Input: part model. Units: mm. Frame: model coordinates. A direction names the side the tool comes from. Round coordinates to 2 decimals unless told otherwise and drop trailing zeros. Loops run counter-clockwise (first coordinate to the right, second up) from the corner with the lowest first, then second, coordinate; pieces in that order, holes last. Notation, with made-up numbers: (-11.5, 87) - (24.5, 87) arc R22 ccw to (24.5, 99) - close; hole circle Ø1 at (57.25, 41.5). An arc over 180 degrees is marked (long way). One line per question, with ' | ' between items. Start each with the question number.
from build123d import *

# Parameters (mm, degrees)
SKETCH1_R           = 6.35
SKETCH1_R_2         = 1.905
SKETCH1_R_3         = 11.43
BOSS_EXTRUDE1_DEPTH = 10.16
SKETCH8_R           = 6.35
CUT_EXTRUDE3_DEPTH  = 9.398
FILLET1_R           = 6.35
FILLET3_R           = 2.54


with BuildPart() as part:
    # Sketch1 → Boss-Extrude1 (new body)
    with BuildSketch(Plane(origin=(0, 0, 0), x_dir=(1, 0, 0), z_dir=(0, 1, 0))):
        with BuildLine():
            ThreePointArc((54.61, -31.75), (22.86, 0), (54.61, 31.75))
            Line((54.61, 31.75), (69.270321928, 31.75))
            ThreePointArc((69.270321928, 31.75), (-76.2, 0), (69.270321928, -31.75))
            Line((69.270321928, -31.75), (54.61, -31.75))
        make_face()
        with Locations(Location((0, -60.96, 0), (0, 0, 270))):
            Circle(SKETCH1_R, mode=Mode.SUBTRACT)
        with Locations(Location((-15.499999988, -15.499999988, 0), (0, 0, 270))):
            Circle(SKETCH1_R_2, mode=Mode.SUBTRACT)
        with Locations(Location((15.499999988, -15.499999988, 0), (0, 0, 270))):
            Circle(SKETCH1_R_2, mode=Mode.SUBTRACT)
        with Locations(Location((-15.499999988, 15.499999988, 0), (0, 0, 270))):
            Circle(SKETCH1_R_2, mode=Mode.SUBTRACT)
        with Locations(Location((0, 0, 0), (0, 0, 270))):
            Circle(SKETCH1_R_3, mode=Mode.SUBTRACT)
        with Locations(Location((15.499999988, 15.499999988, 0), (0, 0, 270))):
            Circle(SKETCH1_R_2, mode=Mode.SUBTRACT)
    extrude(amount=BOSS_EXTRUDE1_DEPTH)

    # Sketch8 → Cut-Extrude3 (cut)
    with BuildSketch(Plane.XZ):
        with BuildLine():
            add(Edge.make_bspline(
                [(27.167528595, 25.920303401), (12.984356547, 19.050000027), (1.04e-07, 19.05)],
                knots=[0, 0, 0, 0.304865692, 0.304865692, 0.304865692], degree=2))
            ThreePointArc((27.167528595, 25.920303401), (42.590415369, 38.092533294), (52.979467942, 54.76875))
            ThreePointArc((52.979467942, 54.76875), (0, 76.2), (-52.979467942, 54.76875))
            add(Edge.make_bspline(
                [(1.04e-07, 19.05), (-29.606058837, 19.049999938), (-52.979467942, 54.76875)],
                knots=[0.304865692, 0.304865692, 0.304865692, 1, 1, 1], degree=2))
        make_face()
        with Locations(Location((0, 60.96, 0), (0, 0, 270))):
            Circle(SKETCH8_R, mode=Mode.SUBTRACT)
    extrude(amount=-CUT_EXTRUDE3_DEPTH, mode=Mode.SUBTRACT)

    # Fillet1
    fillet1_edges = [part.edges().sort_by_distance(p)[0] for p in [
        (69.270321928, 5.08, -31.75),
        (69.270321928, 5.08, 31.75),
    ]]
    fillet(fillet1_edges, radius=FILLET1_R)

    # Fillet3
    # the kernel refuses this fillet: 2.54 mm, written as the material it takes off along each edge
    with BuildSketch(Plane(origin=(54.61, 10.16, -31.75), x_dir=(0, 0, -1), z_dir=(1, 0, 0))) as fillet3_piece_1:
        with BuildLine():
            CenterArc((FILLET3_R, -FILLET3_R), FILLET3_R, 90, 90)
            Line((0, -FILLET3_R), (0, 0))
            Line((0, 0), (FILLET3_R, 0))
        make_face()
    extrude(amount=3.934107304, mode=Mode.SUBTRACT)
    with BuildSketch(Plane(origin=(58.544107304, 10.16, -38.1), x_dir=(0, 0, 1), z_dir=(-1, 0, 0))) as fillet3_piece_2:
        with BuildLine():
            CenterArc((6.35 - FILLET3_R, -FILLET3_R), FILLET3_R, 0, 90)
            Line((6.35, -FILLET3_R), (6.35, 0))
            Line((6.35, 0), (6.35 - FILLET3_R, 0))
        make_face()
    revolve(axis=Axis((58.544107304, 10.16, -38.1), (0, 1, 0)), revolution_arc=123.055731151, mode=Mode.SUBTRACT)
    with BuildSketch(Plane(origin=(0, 10.16, 0), x_dir=(0.8381404052084442, 0, -0.5454545454545454), z_dir=(0.5454545454545454, 0, 0.8381404052084442))) as fillet3_piece_3:
        with BuildLine():
            CenterArc((76.2 - FILLET3_R, -FILLET3_R), FILLET3_R, 0, 90)
            Line((76.2, -FILLET3_R), (76.2, 0))
            Line((76.2, 0), (76.2 - FILLET3_R, 0))
        make_face()
    revolve(axis=Axis((0, 10.16, 0), (0, 1, 0)), revolution_arc=293.888537698, mode=Mode.SUBTRACT)
    with BuildSketch(Plane(origin=(58.544107304, 10.16, 38.1), x_dir=(0, 0, -1), z_dir=(-1, 0, 0))) as fillet3_piece_4:
        with BuildLine():
            CenterArc((6.35 - FILLET3_R, FILLET3_R), FILLET3_R, 270, 90)
            Line((6.35 - FILLET3_R, 0), (6.35, 0))
            Line((6.35, 0), (6.35, FILLET3_R))
        make_face()
    revolve(axis=Axis((58.544107304, 10.16, 38.1), (0, -1, 0)), revolution_arc=123.055731151, mode=Mode.SUBTRACT)
    with BuildSketch(Plane(origin=(58.544107304, 10.16, 31.75), x_dir=(0, -1, 0), z_dir=(-1, 0, 0))) as fillet3_piece_5:
        with BuildLine():
            CenterArc((FILLET3_R, FILLET3_R), FILLET3_R, 180, 90)
            Line((0, FILLET3_R), (0, 0))
            Line((0, 0), (FILLET3_R, 0))
        make_face()
    extrude(amount=3.934107304, mode=Mode.SUBTRACT)
    with BuildSketch(Plane(origin=(54.61, 10.16, 0), x_dir=(0, 0, 1), z_dir=(1, 0, 0))) as fillet3_piece_6:
        with BuildLine():
            CenterArc((31.75 + FILLET3_R, FILLET3_R), FILLET3_R, 180, 90)
            Line((31.75 + FILLET3_R, 0), (31.75, 0))
            Line((31.75, 0), (31.75, FILLET3_R))
        make_face()
    revolve(axis=Axis((54.61, 10.16, 0), (0, -1, 0)), revolution_arc=180, mode=Mode.SUBTRACT)


solid = part.part
(1) Pull-direction query (Z, two-part tool) for faces 4 (the face through (64.171, 3.863, -35.157)), 5 (the face through (-22, 10.16, -1)), 6 (the face through (-47.1, 3.8, -59.9)); classes: released by +Z, released by -Z, zero draft, split by the parting line, or undercut.
(2) Section B-B, the plane y = 5. Give the number of separate pieces and of enclosed holes in the cut face, plus the area to 3 significant figures.
(3) Reachability of faces 1 (the face through (-13.61, 5.01, -15.75)), 2 (the face through (42.41, 4.63, 37.89)), 3 (the face through (57, 4, -31.75)) from +Z, -Z, +X, -X, +Y, -Y: full face, straight path, thin tool, end or side. Return the list, or none.
(4) Pin query (flat end, axial travel): P1, Ø1.5, axis at x = -32.5, z = -25.5, coming from the -Y side; P2, Ø3, axis at x = 24.5, y = 7.5, coming from the +Z side; P3, Ø3.5, axis at x = 15.5, z = 15.5, coming from the +Y side; P4, Ø2, axis at x = 56, y = 5.5, coming from the -Z side. Return the tip coordinate at first contact, or that it passes through.
(5) Line query: line 1 along X through (y, z) = (3.25, 15.5) (3 decimals); line 2 along X through (y, z) = (7.5, 0.5); line 3 along Z through (x, y) = (56.5, 1). Output: solid intervals per line, ascending. Write a range as from..to.
(6) Section A-A, the plane z = 0. Output: boundary loops of the cut face in (x, y), plus the area to 3 significant figures.
Derived:
1) face 4: undercut | face 5: zero draft | face 6: split by the parting line
2) separate pieces: 1 | enclosed holes: 5 | area: 10,700 mm²
3) face 1: +Y, -Y | face 2: +Z, -Y | face 3: +X, +Y, -Y
4) P1: stops at y = 0 | P2: stops at z = 25.37 | P3: passes through | P4: stops at z = -52.74
5) line 1: x = -74.607..-17.405, -13.595..13.595, 17.405..26.901 | line 2: x = -76.2..-11.42, 11.42..22.86 | line 3: z = -51.13..-31.75, 31.75..51.13
6) outline: (-76.2, 0) - (-11.43, 0) - (-11.43, 10.16) - (-73.66, 10.16) arc R2.54 ccw to (-76.2, 7.62) - close; (11.43, 0) - (22.86, 0) - (22.86, 7.62) arc R2.54 ccw to (20.32, 10.16) - (11.43, 10.16) - close | area: 771 mm²
